from build123d import *

# Parameters (mm, degrees)
SALIENTE_EXTRUIR5_DEPTH = 7
CROQUIS5_R              = 1.55
CORTAR_EXTRUIR1_DEPTH   = 71.562029449
SALIENTE_EXTRUIR7_DEPTH = 7
CORTAR_EXTRUIR2_DEPTH   = 74.002747576


with BuildPart() as part:
    # Croquis1 → Saliente-Extruir5 (new body)
    with BuildSketch(Plane.XY):
        with BuildLine():
            Line((-20.5, 30), (-30.5, 30))
            ThreePointArc((-30.5, 30), (-31.232233047, 28.232233047), (-33, 27.5))
            Line((-33, 27.5), (-33, -27.5))
            ThreePointArc((-33, -27.5), (-31.232233047, -28.232233047), (-30.5, -30))
            Line((-30.5, -30), (30.5, -30))
            ThreePointArc((30.5, -30), (31.232233047, -28.232233047), (33, -27.5))
            Line((33, -27.5), (33, 27.5))
            ThreePointArc((33, 27.5), (31.232233047, 28.232233047), (30.5, 30))
            Line((30.5, 30), (20.5, 30))
            Line((20.5, 30), (20.5, 16))
            Line((20.5, 16), (-20.5, 16))
            Line((-20.5, 16), (-20.5, 30))
        make_face()
        with BuildLine():
            Line((-9.486832981, 30), (-20.5, 30))
            Line((-20.5, 30), (-20.5, 16))
            Line((-20.5, 16), (20.5, 16))
            Line((20.5, 16), (20.5, 30))
            Line((20.5, 30), (9.486832981, 30))
            ThreePointArc((9.486832981, 30), (0, 25), (-9.486832981, 30))
        make_face()
        with BuildLine():
            ThreePointArc((-33, 27.5), (-34.767766953, 31.767766953), (-30.5, 30))
            Line((-30.5, 30), (-20.5, 30))
            Line((-20.5, 30), (-20.5, 39))
            Line((-20.5, 39), (-41, 39))
            Line((-41, 39), (-41, -39))
            Line((-41, -39), (41, -39))
            Line((41, -39), (41, 39))
            Line((41, 39), (20.5, 39))
            Line((20.5, 39), (20.5, 30))
            Line((20.5, 30), (30.5, 30))
            ThreePointArc((30.5, 30), (33, 32.5), (35.5, 30))
            ThreePointArc((35.5, 30), (34.767766953, 28.232233047), (33, 27.5))
            Line((33, 27.5), (33, -27.5))
            ThreePointArc((33, -27.5), (34.767766953, -28.232233047), (35.5, -30))
            ThreePointArc((35.5, -30), (33, -32.5), (30.5, -30))
            Line((30.5, -30), (-30.5, -30))
            ThreePointArc((-30.5, -30), (-34.767766953, -31.767766953), (-33, -27.5))
            Line((-33, -27.5), (-33, 27.5))
        make_face()
        with BuildLine():
            Line((-20.5, 57), (-20.5, 39))
            Line((-20.5, 39), (-11.22497216, 39))
            ThreePointArc((-11.22497216, 39), (0, 48), (11.22497216, 39))
            Line((11.22497216, 39), (20.5, 39))
            Line((20.5, 39), (20.5, 57))
            Line((20.5, 57), (-20.5, 57))
        make_face()
        with BuildLine():
            Line((-20.5, 39), (-20.5, 30))
            Line((-20.5, 30), (-9.486832981, 30))
            ThreePointArc((-9.486832981, 30), (-11.291355899, 34.319339102), (-11.22497216, 39))
            Line((-11.22497216, 39), (-20.5, 39))
        make_face()
        with BuildLine():
            ThreePointArc((11.5, 36.5), (10.985185007, 33.097690437), (9.486832981, 30))
            Line((9.486832981, 30), (20.5, 30))
            Line((20.5, 30), (20.5, 39))
            Line((20.5, 39), (11.22497216, 39))
            ThreePointArc((11.22497216, 39), (11.431036258, 37.757541283), (11.5, 36.5))
        make_face()
    extrude(amount=SALIENTE_EXTRUIR5_DEPTH)

    # Croquis5 → Cortar-Extruir1 (cut, through all)
    with BuildSketch(Plane.XY.offset(7)):
        with Locations((-15.5, 52)):
            Circle(CROQUIS5_R)
        with Locations((15.5, 52)):
            Circle(CROQUIS5_R)
        with Locations((15.5, 21)):
            Circle(CROQUIS5_R)
        with Locations((-15.5, 21)):
            Circle(CROQUIS5_R)
    extrude(amount=-CORTAR_EXTRUIR1_DEPTH, mode=Mode.SUBTRACT)

    # Croquis6 → Saliente-Extruir7 (add, through all)
    with BuildSketch(Plane.XY.offset(7)):
        Polygon((-41, 17.857864376), (-41, 36), (-45.071067812, 31.928932188), (-45.071067812, 21.928932188), align=None)
        Polygon((-20.5, 43.242640687), (-24.742640687, 39), (-20.5, 39), align=None)
        Polygon((20.5, 43.242640687), (20.5, 39), (24.742640687, 39), align=None)
        Polygon((45.071067812, 31.928932188), (41, 36), (41, 17.857864376), (45.071067812, 21.928932188), align=None)
        Polygon((41, -21.928932188), (41, -39), (44.535533906, -35.464466094), (44.535533906, -25.464466094), align=None)
        Polygon((41, -39), (23.928932188, -39), (27.464466094, -42.535533906), (37.464466094, -42.535533906), align=None)
        Polygon((-41, -39), (-41, -21.928932188), (-44.535533906, -25.464466094), (-44.535533906, -35.464466094), align=None)
        Polygon((-23.928932188, -39), (-41, -39), (-37.464466094, -42.535533906), (-27.464466094, -42.535533906), align=None)
    extrude(amount=-SALIENTE_EXTRUIR7_DEPTH)

    # Croquis7 → Cortar-Extruir2 (cut, through all)
    with BuildSketch(Plane.XY.offset(7)):
        Polygon((-20.5, 52.757359313), (-16.257359313, 57), (-20.5, 57), align=None)
        Polygon((20.5, 57), (16.257359313, 57), (20.5, 52.757359313), align=None)
        Polygon((-41, 39), (-41, 36), (-38, 39), align=None)
        Polygon((38, 39), (41, 36), (41, 39), align=None)
    extrude(amount=-CORTAR_EXTRUIR2_DEPTH, mode=Mode.SUBTRACT)


solid = part.part
Model file for the job. Use its own axes, mm. A direction names the side the tool comes from. Coordinates: 2 decimals unless noted, no trailing zeros. Order: outer loops, then holes, each group sorted by start corner. A loop starts at its lowest first (then second) coordinate and runs counter-clockwise, first axis right, second up. Notation, with made-up numbers: (41.5, -1) -> (73.5, -1) arc R14 cw to (73.5, 24) -> close; hole circle Ø5 at (84, 47). An arc over 180 degrees is marked (long way). Return JSON: item names as keys, results as strings. Group by question number.
Item 1: Flat gauge pins, fed straight in: P1, Ø3.5, axis at y = 49, z = 5, coming from the -X side; P2, Ø3, axis at x = 10.5, z = 2, coming from the -Y side; P3, Ø2, axis at y = 6.5, z = 2.5, coming from the -X side; P4, Ø5, axis at x = 15.5, y = 52, coming from the +Z side. Where does each tip first touch, or does it go through?
Item 2: Saw through at B-B on z = 5.25. State how many separate pieces and enclosed holes the cut face has, then the cut area to 3 significant figures.
Item 3: Saw through at A-A on x = -3. Write the cut outline in (y, z).
Item 4: Wall check: line 1 along Y through (x, z) = (-15.5, 2); line 2 along X through (y, z) = (30, 2.25); line 3 along Y through (x, z) = (-33, 5.5). Give the ranges that are in metal, low to high. Write a range as [from, to].
Item 5: Pull direction Y, two halves, no side cores. Call faces 1 (the flat face through (43.007, 19.865, 3.549)), 2 (the cylindrical face through (-15.702, 22.537, 3.549)), 3 (the flat face through (25.67, -40.74, 3.55)), 4 (the flat face through (-20.5, 48, 3)): pulls with the +Y half, pulls with the -Y half, needs draft (parallel to the pull), parting line crosses it, or undercut.
Item 6: Tool access for faces 5 (the flat face through (41, -2, 3)), 6 (the flat face through (-43.06, 19.92, 3.55)), 7 (the flat face through (0, -39, 3)), 8 (the flat face through (-44.536, -30, 4)): list every direction of +Z, -Z, +X, -X, +Y, -Y with a clear straight run to the whole face (end or side of a thin tool).
Item 7: Saw through at D-D on y = -24. Write the cut outline in (x, z).
Item 8: Saw through at C-C on y = 0. Write the cut outline in (x, z).
Values found:
{
 "1": {"P1": "stops at x = -20.5", "P2": "stops at y = -39", "P3": "stops at x = -41", "P4": "stops at z = 7"},
 "2": {"separate pieces": "1", "enclosed holes": "9", "area": "6,910 mm2"},
 "3": {"outline": "(-39, 0) -> (25.4, 0) -> (25.4, 7) -> (-39, 7) -> close; (47.6, 0) -> (57, 0) -> (57, 7) -> (47.6, 7) -> close"},
 "4": {"line 1": "y = [-39, 19.45], [22.55, 50.45], [53.55, 57]", "line 2": "x = [-45.07, -35.5], [-30.5, -9.49], [9.49, 30.5], [35.5, 45.07]", "line 3": "y = [-42.54, -32.5], [-27.5, 27.5], [32.5, 39]"},
 "5": {"face 1": "undercut", "face 2": "undercut", "face 3": "pulls with the -Y half", "face 4": "needs draft"},
 "6": {"face 5": "+Z, -Z, +X", "face 6": "+Z, -Z, -X", "face 7": "+Z, -Z, -Y", "face 8": "+Z, -Z, -X, -Y"},
 "7": {"outline": "(-43.07, 0) -> (43.07, 0) -> (43.07, 7) -> (-43.07, 7) -> close"},
 "8": {"outline": "(-41, 0) -> (41, 0) -> (41, 7) -> (-41, 7) -> close"}
}
